Can you work these out from the model? Positions are in its coordinate system, mm. A direction names the side the tool comes from. Coordinates: 2 decimals unless noted, no trailing zeros. Order: outer loops, then holes, each group sorted by start corner. A loop starts at its lowest first (then second) coordinate and runs counter-clockwise, first axis right, second up. Notation, with made-up numbers: M -26.5,42 L 23.5,42 A17 ccw 23.5,67 Z; hole C 34.25,-29.5 d3. An arc over 180 degrees is marked long. Answer as CSV lines item,"result". Start each with the question number.
1. If we section it at D-D (y = 32.5): List the corners of the cut face in (x, z) for me.
2. On a 3-axis mill with a long thin cutter (end or side, diameter ignored), from which of +Z, -Z, +X, -X, +Y, -Y can I reach the whole of each face in a straight line? I mean faces 4 (the face through (-5.29, 4.93, 175.48)), 5 (the face through (-11, 30, 163)), 6 (the face through (-5, 47, 174)). Say none if no direction works.
3. If we mould it in two halves opening along Z, with no side actions, what happens to faces 1 (the face through (-24, 32, 184.16)), 2 (the face through (-11, 10, 169)), 3 (the face through (-5, 10, 174))? For each: released by +Z, released by -Z, zero draft, split by the parting line, or undercut.
4. If we section it at C-C (x = -18): List the corners of the cut face in (y, z) for me.
5. If we section it at B-B (z = 157): List the corners of the cut face in (x, y) for me.
6. Will these pins go through, and if not, where does the flat tip stop? pin 1 (3 mm diameter, centred on y = 36, z = 167.5, fed in from -X); pin 2 (22 mm diameter, centred on y = 15.5, z = 165.5, fed in from -X); pin 3 (3.5 mm diameter, centred on x = 5, z = 143.16, fed in from -Y).
7. I need wall thicknesses on line 1 along Z through (x, y) = (-5, 3); line 2 along Z through (x, y) = (7, 36); line 3 along X through (y, z) = (11, 165). Which ranges of each line are inside material? Lowest first, please. Write a range as from..to.
8. If we section it at A-A (y = 39): List the corners of the cut face in (x, z) for me, plus the area to 3 significant figures.
```python
from build123d import *

# Parameters (mm, degrees)
EXTRUDE_1_DEPTH       = 172
SHELL_START           = 6
SHELL_1_DEPTH         = 160
SKETCH_2_W            = 36
SKETCH_2_H            = 16
CUT_EXTRUDE_1_DEPTH   = 74
EXTRUDE_2_DEPTH       = 2
SKETCH_4_R            = 10
CUT_EXTRUDE_2_DEPTH   = 186
SKETCH_5_R            = 1.5
CUT_EXTRUDE_3_DEPTH   = 10
EXTRUDE_3_DEPTH       = 172
SKETCH_7_W            = 36
SKETCH_7_H            = 16
CUT_EXTRUDE_4_DEPTH   = 172
SKETCH_8_W            = 6
SKETCH_8_H            = 172
CUT_EXTRUDE_5_DEPTH   = 3
EXTRUDE_4_DEPTH       = 15
CHAMFER_1_SIZE        = 15
CHAMFER_2_SIZE        = 15
CHAMFER_3_SIZE        = 8
SKETCH_10_R           = 1.35
CUT_EXTRUDE_6_DEPTH   = 15
SKETCH_12_R           = 1.35
CUT_EXTRUDE_7_DEPTH   = 15
SKETCH_14_OUTSIDE_W   = 213.548
SKETCH_14_OUTSIDE_H   = 97.548
SKETCH_14_OUTSIDE_W_2 = 15
SKETCH_14_OUTSIDE_H_2 = 56
CUT_EXTRUDE_8_DEPTH   = 82.5
EXTRUDE_5_DEPTH       = 15
CUT_EXTRUDE_9_DEPTH   = 15
SKETCH_17_W           = 13
SKETCH_17_H           = 5
EXTRUDE_6_DEPTH       = 15
EXTRUDE_7_DEPTH       = 20
SHELL_START_2         = 78.159554327
SHELL_2_DEPTH         = 10
EXTRUDE_8_DEPTH       = 28
CUT_EXTRUDE_10_DEPTH  = 20
CUT_EXTRUDE_11_DEPTH  = 20
SKETCH_23_R           = 1.65
SKETCH_23_R_2         = 1.35
CUT_EXTRUDE_12_DEPTH  = 22
SKETCH_26_R           = 1.35
CUT_EXTRUDE_14_DEPTH  = 10
CUT_EXTRUDE_15_DEPTH  = 82.5


# Read off the part's stored shape, not the designer's step: 抽壳1, 抽壳2
with BuildPart() as part:
    # 草图1 → 凸台-拉伸1 (new body)
    with BuildSketch(Plane.XY):
        with BuildLine():
            Line((0, 0), (0, 40))
            Line((0, 40), (-5, 40))
            Line((-5, 40), (-5, 53))
            Line((-5, 53), (-23, 53))
            Line((-23, 53), (-64.888578151, 47.050698608))
            Line((-64.888578151, 47.050698608), (-15.121320344, -2.121320344))
            ThreePointArc((-15.121320344, -2.121320344), (-14.148050297, -2.771638598), (-13, -3))
            Line((-13, -3), (-5, -3))
            Line((-5, -3), (-5, 0))
            Line((-5, 0), (0, 0))
        make_face()
    extrude(amount=EXTRUDE_1_DEPTH)

    # 抽壳1 outline → 抽壳1 (cut)
    with BuildSketch(Plane.XY.offset(SHELL_START)):
        Polygon((-11, 6), (-6, 6), (-6, 34), (-11, 34), (-11, 47), (-22.576046832, 47), (-52.061983815, 42.812206246), (-11.767841448, 3), (-11, 3), align=None)
    extrude(amount=SHELL_1_DEPTH, mode=Mode.SUBTRACT)

    # 草图2 → 切除-拉伸1 (cut)
    with BuildSketch(Plane(origin=(0, 0, 0), x_dir=(0, 0, -1), z_dir=(1, 0, 0))):
        with Locations((-136, 10)):
            Rectangle(SKETCH_2_W, SKETCH_2_H)
        with Locations((-36, 10)):
            Rectangle(SKETCH_2_W, SKETCH_2_H)
    extrude(amount=-CUT_EXTRUDE_1_DEPTH, mode=Mode.SUBTRACT)

    # 草图3 → 凸台-拉伸2 (add, symmetric)
    with BuildSketch(Plane(origin=(0, 0, 86), x_dir=(-1, 0, 0), z_dir=(0, 0, -1))):
        Polygon((5, 53), (5, 40), (0, 40), (0, 0), (5, 0), (5, -3), (13, -3), (16.579355858, -0.680723591), (64.888578151, 47.050698608), (23, 53), align=None)
    extrude(amount=EXTRUDE_2_DEPTH, both=True)

    # 草图4 → 切除-拉伸2 (cut)
    with BuildSketch(Plane.XY.offset(172)):
        with Locations((-15, 21.071297481)):
            Circle(SKETCH_4_R)
    extrude(amount=-CUT_EXTRUDE_2_DEPTH, mode=Mode.SUBTRACT)

    # 草图5 → 切除-拉伸3 (cut)
    with BuildSketch(Plane(origin=(0, 53, 0), x_dir=(1, 0, 0), z_dir=(0, 1, 0))):
        with Locations(Location((-13.338195438, -63.5, 0), (0, 0, 270))):
            Circle(SKETCH_5_R)
        with Locations(Location((-13.338195438, -108.5, 0), (0, 0, 270))):
            Circle(SKETCH_5_R)
    extrude(amount=-CUT_EXTRUDE_3_DEPTH, mode=Mode.SUBTRACT)

    # 草图6 → 凸台-拉伸3 (add)
    with BuildSketch(Plane.XY.offset(172)):
        Polygon((-11, 6), (-14.804157153, 6), (-11.767841448, 3), (-11, 3), align=None)
    extrude(amount=-EXTRUDE_3_DEPTH)

    # 草图7 → 切除-拉伸4 (cut)
    with BuildSketch(Plane(origin=(0, 0, 0), x_dir=(0, 0, -1), z_dir=(1, 0, 0))):
        with Locations((-136, 10)):
            Rectangle(SKETCH_7_W, SKETCH_7_H)
        with Locations((-36, 10)):
            Rectangle(SKETCH_7_W, SKETCH_7_H)
    extrude(amount=-CUT_EXTRUDE_4_DEPTH, mode=Mode.SUBTRACT)

    # 草图8 → 切除-拉伸5 (cut)
    with BuildSketch(Plane.XZ.offset(3)):
        with Locations((-8, 86)):
            Rectangle(SKETCH_8_W, SKETCH_8_H)
    extrude(amount=-CUT_EXTRUDE_5_DEPTH, mode=Mode.SUBTRACT)

    # 草图9 → 凸台-拉伸4 (add)
    with BuildSketch(Plane(origin=(0, 0, 0), x_dir=(0, 0, -1), z_dir=(1, 0, 0))):
        Polygon((-86, 40), (-151, 40), (-151, 35), (-86, 35), (-21, 35), (-21, 40), align=None)
    extrude(amount=EXTRUDE_4_DEPTH)

    # 倒角1
    chamfer_1_edges = [part.edges().sort_by_distance(p)[0] for p in [
        (15, 37.5, 151),
    ]]
    chamfer(chamfer_1_edges, length=CHAMFER_1_SIZE - 0.0001)  # a hair under: the kernel refuses the full size

    # 倒角2
    chamfer_2_edges = [part.edges().sort_by_distance(p)[0] for p in [
        (15, 37.5, 21),
    ]]
    chamfer(chamfer_2_edges, length=CHAMFER_2_SIZE - 0.0001)  # a hair under: the kernel refuses the full size

    # 倒角3
    chamfer_3_edges = [part.edges().sort_by_distance(p)[0] for p in [
        (0, 35, 86),
    ]]
    chamfer(chamfer_3_edges, length=CHAMFER_3_SIZE)

    # 草图10 → 切除-拉伸6 (cut)
    with BuildSketch(Plane.XZ):
        with Locations((-5, 158)):
            Circle(SKETCH_10_R)
        with Locations((-5, 111)):
            Circle(SKETCH_10_R)
        with Locations((-5, 61)):
            Circle(SKETCH_10_R)
        with Locations((-5, 14.01360213)):
            Circle(SKETCH_10_R)
    extrude(amount=-CUT_EXTRUDE_6_DEPTH, mode=Mode.SUBTRACT)

    # 草图12 → 切除-拉伸7 (cut)
    with BuildSketch(Plane(origin=(0, 40, 0), x_dir=(1, 0, 0), z_dir=(0, 1, 0))):
        with Locations(Location((5, -41, 0), (0, 0, 270))):
            Circle(SKETCH_12_R)
        with Locations(Location((5, -86, 0), (0, 0, 270))):
            Circle(SKETCH_12_R)
        with Locations(Location((5, -131, 0), (0, 0, 270))):
            Circle(SKETCH_12_R)
    extrude(amount=-CUT_EXTRUDE_7_DEPTH, mode=Mode.SUBTRACT)

    # 草图14 outside → 切除-拉伸8 (cut, symmetric)
    with BuildSketch(Plane(origin=(0, 0, 0), x_dir=(0, 0, -1), z_dir=(1, 0, 0))):
        with Locations((-86, 25)):
            Rectangle(SKETCH_14_OUTSIDE_W, SKETCH_14_OUTSIDE_H)
        with Locations((-75.659554327, 25)):
            Rectangle(SKETCH_14_OUTSIDE_W_2, SKETCH_14_OUTSIDE_H_2, mode=Mode.SUBTRACT)
    extrude(amount=CUT_EXTRUDE_8_DEPTH, both=True, mode=Mode.SUBTRACT)

    # 草图15 → 凸台-拉伸5 (add)
    with BuildSketch(Plane(origin=(0, 0, 68.159554327), x_dir=(-1, 0, 0), z_dir=(0, 0, -1))):
        Polygon((0, 0), (-2, 0), (-2, 29), (0, 27), align=None)
    extrude(amount=-EXTRUDE_5_DEPTH)

    # 草图16 → 切除-拉伸9 (cut)
    with BuildSketch(Plane(origin=(0, 0, 68.159554327), x_dir=(-1, 0, 0), z_dir=(0, 0, -1))):
        Polygon((-2, 29), (-2, 35), (-8, 35), align=None)
    extrude(amount=-CUT_EXTRUDE_9_DEPTH, mode=Mode.SUBTRACT)

    # 草图17 → 凸台-拉伸6 (add)
    with BuildSketch(Plane(origin=(0, 0, 68.159554327), x_dir=(-1, 0, 0), z_dir=(0, 0, -1))):
        with Locations((-8.5, 32.5)):
            Rectangle(SKETCH_17_W, SKETCH_17_H)
    extrude(amount=-EXTRUDE_6_DEPTH)

    # 草图18 → 凸台-拉伸7 (add)
    with BuildSketch(Plane(origin=(0, 0, 68.159554327), x_dir=(-1, 0, 0), z_dir=(0, 0, -1))):
        with BuildLine():
            Line((-15, 40), (-15, 30))
            Line((-15, 30), (-2, 30))
            Line((-2, 30), (-2, 0))
            Line((-2, 0), (11, 0))
            Line((11, 0), (11, -3))
            Line((11, -3), (13, -3))
            ThreePointArc((13, -3), (14.148050297, -2.771638598), (15.121320344, -2.121320344))
            Line((15.121320344, -2.121320344), (64.888578151, 47.050698608))
            Line((64.888578151, 47.050698608), (23, 53))
            Line((23, 53), (5, 53))
            Line((5, 53), (5, 40))
            Line((5, 40), (-15, 40))
        make_face()
    extrude(amount=-EXTRUDE_7_DEPTH)

    # 抽壳2 outline → 抽壳2 (cut)
    with BuildSketch(Plane.XY.offset(SHELL_START_2)):
        Polygon((-8, 30), (-15, 30), (-15, 43), (-22.293411387, 43), (-43.510920925, 39.986544671), (-13.161382076, 10), (-8, 10), align=None)
    extrude(amount=SHELL_2_DEPTH, mode=Mode.SUBTRACT)

    # 草图20 → 凸台-拉伸8 (add)
    with BuildSketch(Plane.XY.offset(88.159554327)):
        Polygon((15, 40), (-15, 40), (-15, 30), (-8, 30), (-8, 22), (2, 22), (2, 30), (15, 30), align=None)
    extrude(amount=EXTRUDE_8_DEPTH)

    # 草图21 → 切除-拉伸10 (cut)
    with BuildSketch(Plane(origin=(2, 0, 0), x_dir=(0, 0, -1), z_dir=(1, 0, 0))):
        Polygon((-116.159554327, 30), (-88.159554327, 22), (-116.159554327, 22), align=None)
    extrude(amount=-CUT_EXTRUDE_10_DEPTH, mode=Mode.SUBTRACT)

    # 草图22 → 切除-拉伸11 (cut)
    with BuildSketch(Plane(origin=(0, 40, 0), x_dir=(1, 0, 0), z_dir=(0, 1, 0))):
        Polygon((-8, -116.159554327), (-15, -116.159554327), (-15, -88.159554327), (-5, -116.159554327), align=None)
    extrude(amount=-CUT_EXTRUDE_11_DEPTH, mode=Mode.SUBTRACT)

    # 草图23 → 切除-拉伸12 (cut)
    with BuildSketch(Plane(origin=(0, 40, 0), x_dir=(1, 0, 0), z_dir=(0, 1, 0))):
        with Locations(Location((7.2, -71.159554327, 0), (0, 0, 270))):
            Circle(SKETCH_23_R)
        with Locations(Location((5, -109.159554327, 0), (0, 0, 270))):
            Circle(SKETCH_23_R_2)
    extrude(amount=-CUT_EXTRUDE_12_DEPTH, mode=Mode.SUBTRACT)

    # 草图26 → 切除-拉伸14 (cut)
    with BuildSketch(Plane.XZ):
        with Locations((-5, 78.159554327)):
            Circle(SKETCH_26_R)
    extrude(amount=-CUT_EXTRUDE_14_DEPTH, mode=Mode.SUBTRACT)


with BuildPart() as body_2:
    # 镜向2: mirrored copy
    add(part.part.mirror(Plane.XY.offset(126.159554327)))


with BuildPart() as part_1:
    add(part.part)

    # 草图27 → 切除-拉伸15 (cut, symmetric)
    with BuildSketch(Plane(origin=(0, 40, 0), x_dir=(1, 0, 0), z_dir=(0, 1, 0))):
        Polygon((-70.30444709, -126.427743847), (59.164340296, -124.069061785), (93.545633321, -94.969295867), (93.545633321, -36.488882893), (-105.077867855, -19.264077709), (-117.933649563, -88.897060516), align=None)
    extrude(amount=CUT_EXTRUDE_15_DEPTH, both=True, mode=Mode.SUBTRACT)


solid = body_2.part
```
Solved:
1,outline,"M -50.16,164.16 L -35.93,164.16 L -35.93,174.16 L -15,174.16 L -15,164.16 L -5,136.16 L 15,136.16 L 15,184.16 L -50.16,184.16 Z; hole C 5,143.16 d2.7; hole C 7.2,181.16 d3.3"
2,face 4,"-Y"
2,face 5,"-Z"
2,face 6,"+Z, -Z, +X, +Y"
3,face 1,"released by +Z"
3,face 2,"zero draft"
3,face 3,"undercut"
4,outline,"M 0.72,164.16 L 14.78,164.16 L 14.78,174.16 L 43,174.16 L 43,164.16 L 53,164.16 L 53,184.16 L 0.72,184.16 Z"
5,outline,"M -12.44,30 L -8,30 L -8,24.05 L 2,24.05 L 2,30 L 15,30 L 15,40 L -12.44,40 Z"
6,pin 1,"x = -55.22"
6,pin 2,"x = -44.09"
6,pin 3,"y = 30"
7,line 1,"164.16..172.81, 175.51..184.16"
7,line 2,"136.16..179.52, 182.8..184.16"
7,line 3,"-28.4..-14.17, -8..2"
8,outline,"M -56.74,164.16 L -42.51,164.16 L -42.51,174.16 L -15,174.16 L -15,164.16 L -5,136.16 L 15,136.16 L 15,184.16 L -56.74,184.16 Z; hole C 5,143.16 d2.7; hole C 7.2,181.16 d3.3"
8,area,"1,850 mm²"
